The figure shows three views and two pictorial views of one solid part (mm, origin at its lowest corner). Answer the questions. A direction names the side the tool comes from. Round coordinates to 2 decimals unless told otherwise and drop trailing zeros. Write each loop counter-clockwise with the first axis right and the second up, starting at its lowest first coordinate (ties: lowest second). Pieces come first, ordered by that corner, then holes. Notation, with made-up numbers: M -14,-38 L -3,-38 A26 cw -3,-21 Z; hole C 21,-10 d11. An arc over 180 degrees is marked long. One line per item, written item: value. Start each with the question number.
Q1. Consider probe 1 along Y at (x, z) = (4.65, 6); probe 2 along Y at (x, z) = (6.4, 6); probe 3 along Y at (x, z) = (6, 9). Determine where each line is inside the solid, lowest interval first.
Q2. Find section C-C (y = 21.1). Write down the section's boundary in (x, z), and give its area (3 significant figures).
Q3. A tool of negligible diameter and unlimited length cuts with its end or side. For the marked faces 1 and 2, from which of +Z, -Z, +X, -X, +Y, -Y can it reach the whole face along a straight path? Write none if from no direction.
Q4. Given pin 1 Ø5 at (x, y) = (9.5, 19.5) entering from +Z; pin 2 Ø5.5 at (y, z) = (22.5, 3.5) entering from -X; pin 3 Ø1.5 at (x, y) = (2, 11.5) entering from +Z, each flat-ended and moving along its own axis, determine where each tip first touches the part or whether it passes through.
Q5. Find section B-B (x = 6). Write down the section's boundary in (y, z), and give its area (3 significant figures).
Q6. The mould has two halves that part along Z. Classify the marked faces 3, 4 and 5: released by +Z, released by -Z, zero draft, split by the parting line, or undercut.
Q7. Find section D-D (y = 15). Write down the section's boundary in (x, z), and give its area (3 significant figures).
Q8. Find section A-A (z = 6). Write down the section's boundary in (x, y), and give its area (3 significant figures).
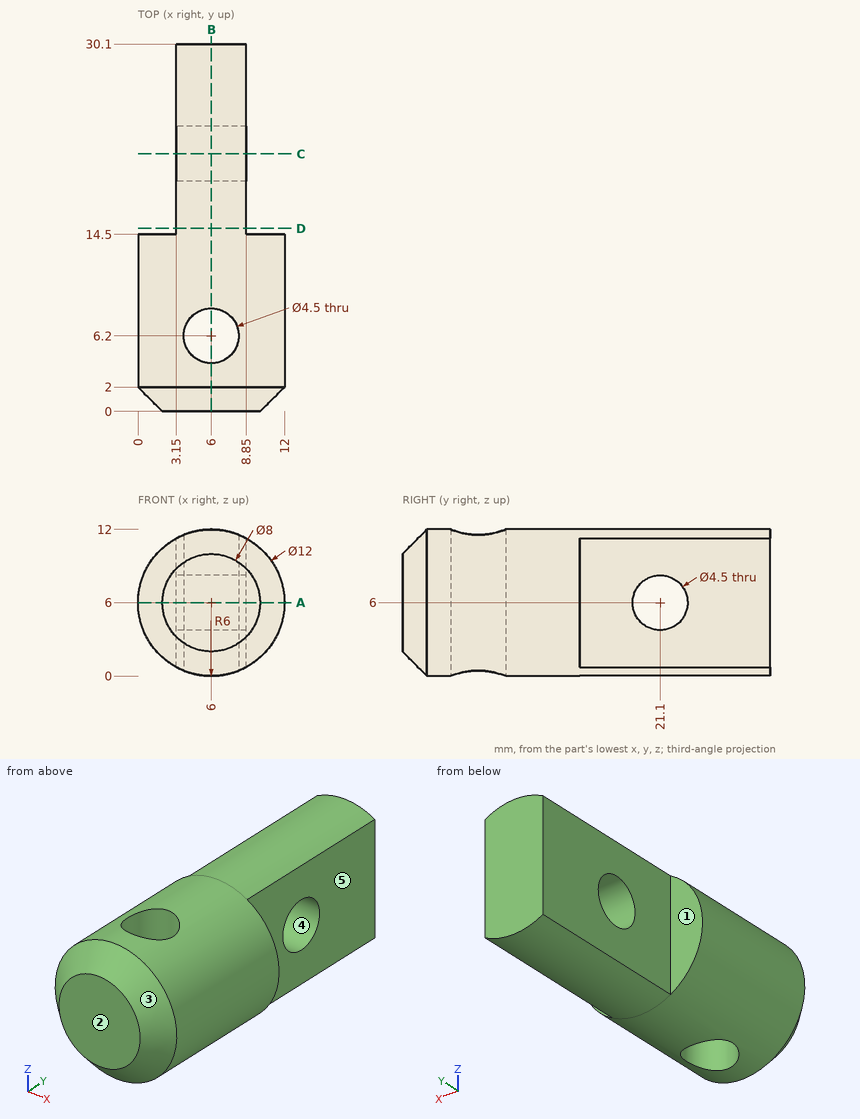
The answers:
1. probe 1: 0 to 4.4, 8 to 18.85, 23.35 to 30.1
1. probe 2: 0 to 3.99, 8.41 to 18.85, 23.35 to 30.1
1. probe 3: 0 to 3.95, 8.45 to 30.1
2. outline: M 3.15,0.72 A6 ccw 8.85,0.72 L 8.85,3.75 L 3.15,3.75 Z; M 3.15,8.25 L 8.85,8.25 L 8.85,11.28 A6 ccw 3.15,11.28 Z
2. area: 40.1 mm2
3. face 1: +Z, -Z, -X, +Y
3. face 2: +Z, -Z, +X, -X, -Y
4. pin 1: z = 11.92
4. pin 2: x = 3.15
4. pin 3: z = 11.04
5. outline: M 0,2 L 2,0 L 3.95,0 L 3.95,12 L 2,12 L 0,10 Z; M 8.45,0 L 30.1,0 L 30.1,12 L 8.45,12 Z; hole C 21.1,6 d4.5
5. area: 287 mm2
6. face 3: split by the parting line
6. face 4: undercut
6. face 5: zero draft
7. outline: M 3.15,0.72 A6 ccw 8.85,0.72 L 8.85,11.28 A6 ccw 3.15,11.28 Z
7. area: 65.7 mm2
8. outline: M 0,2 L 2,0 L 10,0 L 12,2 L 12,14.5 L 8.85,14.5 L 8.85,18.85 L 3.15,18.85 L 3.15,14.5 L 0,14.5 Z; M 3.15,23.35 L 8.85,23.35 L 8.85,30.1 L 3.15,30.1 Z; hole C 6,6.2 d4.5
8. area: 217 mm2
